Part print with two shaded views. Sizes in mm from the minimum x, y, z corner. Give positions to 0.01 mm unless a question says otherwise; leave off trailing zeros. Order: outer loops, then holes, each group sorted by start corner. A loop starts at its lowest first (then second) coordinate and runs counter-clockwise, first axis right, second up. Notation, with made-up numbers: (28, 24) -> (66, 24) arc R21 cw to (66, 49) -> close; hole circle Ø8 at (82, -29). An arc over 180 degrees is marked (long way). Write item = value, one per line. Start each with the question number.
Item 1: Band-saw the part on C-C on z = 1. Write the cut outline in (x, y), plus the area to 3 significant figures.
Item 2: Drill centre lines: line 1 along Z through (x, y) = (2, 5); line 2 along Y through (x, z) = (2.35, 5); line 3 along Z through (x, y) = (2, 7). Where is each one in solid material? Low to high.
Item 3: Band-saw the part on A-A on y = 5. Write the cut outline in (x, z), plus the area to 3 significant figures.
Item 4: Band-saw the part on D-D on x = 0.4. Write the cut outline in (y, z), plus the area to 3 significant figures.
Item 5: Band-saw the part on B-B on z = 5. Write the cut outline in (x, y), plus the area to 3 significant figures.
Item 6: Pull direction Z, two halves, no side cores. Call the marked faces 1, 2, 3 and 4: +Z half, -Z half, draft (parallel to the pull), parting line (faces both ways), or undercut.
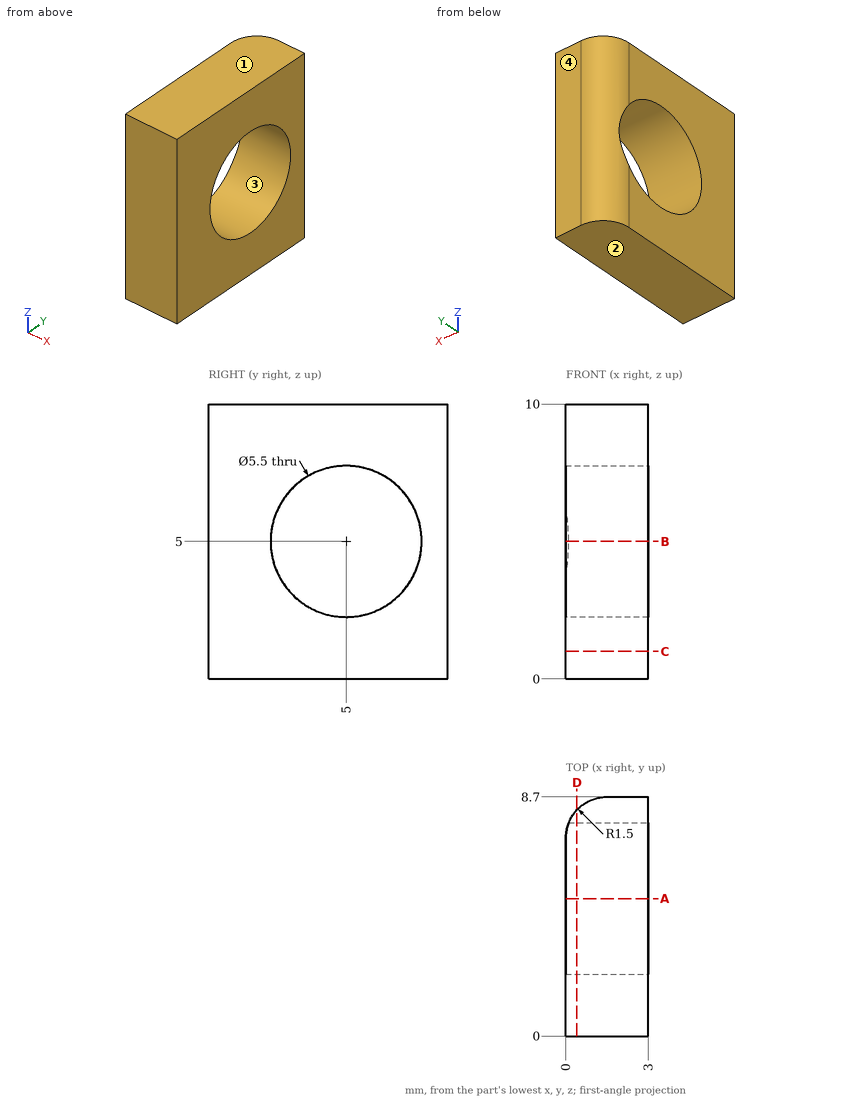
Values found:
q1.outline = (0, 0) -> (3, 0) -> (3, 8.7) -> (1.5, 8.7) arc R1.5 ccw to (0, 7.2) -> close
q1.area = 25.6 mm^2
q2.line_1 = 0 to 2.25, 7.75 to 10
q2.line_2 = 0 to 2.25, 7.75 to 8.7
q2.line_3 = 0 to 3.11, 6.89 to 10
q3.outline = (0, 0) -> (3, 0) -> (3, 2.25) -> (0, 2.25) -> close; (0, 7.75) -> (3, 7.75) -> (3, 10) -> (0, 10) -> close
q3.area = 13.5 mm^2
q4.outline = (0, 0) -> (8.22, 0) -> (8.22, 10) -> (0, 10) -> close; hole circle Ø5.5 at (5, 5)
q4.area = 58.4 mm^2
q5.outline = (0, 0) -> (3, 0) -> (3, 2.25) -> (0, 2.25) -> close; (0.1, 7.75) -> (3, 7.75) -> (3, 8.7) -> (1.5, 8.7) arc R1.5 ccw to start
q5.area = 9.14 mm^2
q6.face_1 = +Z half
q6.face_2 = -Z half
q6.face_3 = undercut
q6.face_4 = draft
